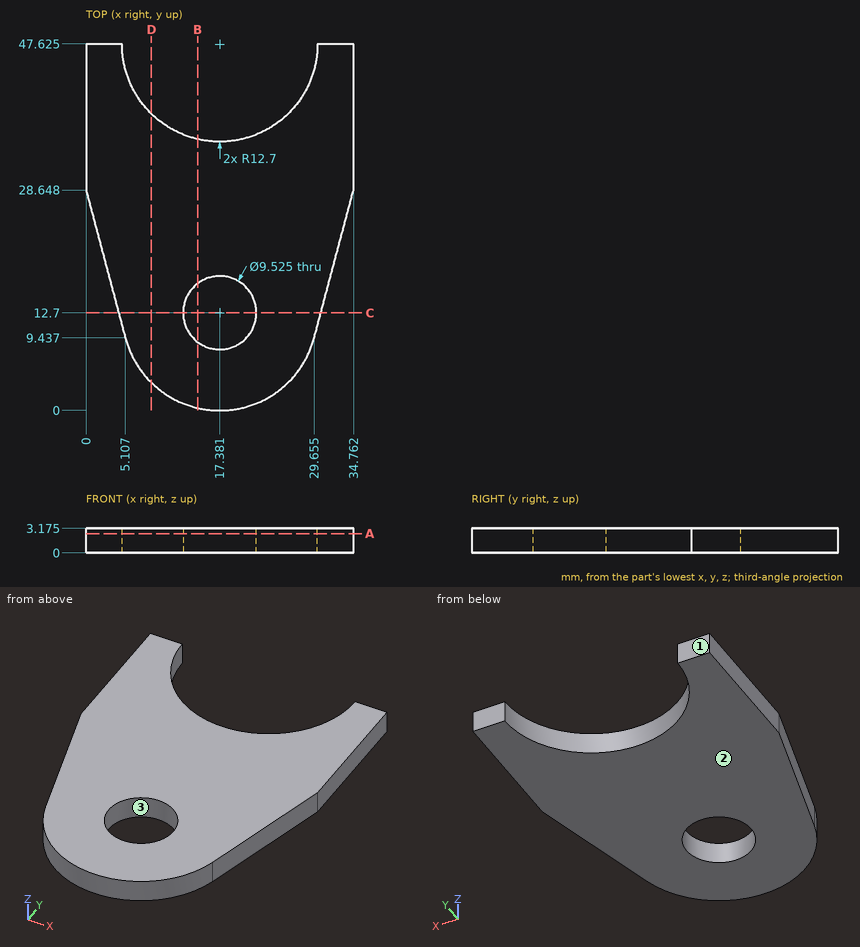
Design review of the part shown in the three views and the two pictorial views. Dimensions are in mm from the part's minimum x, y and z. Round coordinates to 2 decimals unless told otherwise and drop trailing zeros. Loops run counter-clockwise (first coordinate to the right, second up) from the corner with the lowest first, then second, coordinate; pieces in that order, holes last. Notation, with made-up numbers: (-2, -36.5) -> (37, -36.5) arc R15 cw to (37, -25.5) -> close; hole circle Ø9 at (26, 68.25). An arc over 180 degrees is marked (long way). Return JSON: item names as keys, results as strings.
(1) For line 1 (Y direction, x = 16.5, z = 0.5) (1 decimal); line 2 (Y direction, x = 14, z = 2.9) (1 decimal); line 3 (X direction, y = 11, z = 1.4), list the stretches that pass through material, from the lowest coordinate up.
Solved:
{"line 1": "0 to 8, 17.4 to 35", "line 2": "0.5 to 9.3, 16.1 to 35.4", "line 3": "4.69 to 12.93, 21.83 to 30.07"}
(2) For pin 1 (1 mm diameter, centred on x = 7.5, z = 0.5, fed in from +Y), flat-tipped, find the tip position at first contact; note if it passes through.
Solved:
{"pin 1": "y = 40.31"}
(3) Add section B-B on x = 14.5. Write out the cut boundary in (y, z) (1 decimal).
Solved:
{"outline": "(0.3, 0) -> (8.9, 0) -> (8.9, 3.2) -> (0.3, 3.2) -> close; (16.5, 0) -> (35.3, 0) -> (35.3, 3.2) -> (16.5, 3.2) -> close"}
(4) Add section D-D on x = 8.5. Write out the cut boundary in (y, z) (1 decimal), plus the area to 3 significant figures.
Solved:
{"outline": "(3.6, 0) -> (38.5, 0) -> (38.5, 3.2) -> (3.6, 3.2) -> close", "area": "111 mm2"}
(5) Add section A-A on z = 2.5. Write out the cut boundary in (x, y) (1 decimal), plus the area to 3 significant figures.
Solved:
{"outline": "(0, 28.6) -> (5.1, 9.4) arc R12.7 ccw to (29.7, 9.4) -> (34.8, 28.6) -> (34.8, 47.6) -> (30.1, 47.6) arc R12.7 cw to (4.7, 47.6) -> (0, 47.6) -> close; hole circle Ø9.5 at (17.4, 12.7)", "area": "1,080 mm2"}
(6) The part is to be moulded in two halves that separate along Y. For the marked faces 1, 2 and 3, say which applies: released by +Y, released by -Y, zero draft, split by the parting line, or undercut.
Solved:
{"face 1": "released by +Y", "face 2": "zero draft", "face 3": "undercut"}
(7) Add section C-C on y = 12.7. Write out the cut boundary in (x, z) (1 decimal).
Solved:
{"outline": "(4.2, 0) -> (12.6, 0) -> (12.6, 3.2) -> (4.2, 3.2) -> close; (22.1, 0) -> (30.5, 0) -> (30.5, 3.2) -> (22.1, 3.2) -> close"}
